```python
from build123d import *

# Parameters (mm, degrees)
SKETCH1_R           = 9
BOSS_EXTRUDE1_DEPTH = 5
CUT_EXTRUDE1_START  = -3.9
SKETCH2_R           = 9
SKETCH2_R_2         = 8
CUT_EXTRUDE1_DEPTH  = 3.9
SKETCH3_R           = 4
CUT_EXTRUDE2_DEPTH  = 5
FILLET1_R           = 0.5
FILLET2_R           = 0.1
FILLET3_R           = 0.1


with BuildPart() as part:
    # Sketch1 → Boss-Extrude1 (new body)
    with BuildSketch(Plane(origin=(0, 0, 0), x_dir=(1, 0, 0), z_dir=(0, 1, 0))):
        with Locations(Location((0, 0, 0), (0, 0, 270))):
            Circle(SKETCH1_R)
    extrude(amount=BOSS_EXTRUDE1_DEPTH)

    # Sketch2 → Cut-Extrude1 (cut)
    with BuildSketch(Plane(origin=(0, 5, 0), x_dir=(1, 0, 0), z_dir=(0, 1, 0)).offset(CUT_EXTRUDE1_START)):
        with Locations(Location((0, 0, 0), (0, 0, 270))):
            Circle(SKETCH2_R)
        with Locations(Location((0, 0, 0), (0, 0, 270))):
            Circle(SKETCH2_R_2, mode=Mode.SUBTRACT)
    extrude(amount=CUT_EXTRUDE1_DEPTH, mode=Mode.SUBTRACT)

    # Sketch3 → Cut-Extrude2 (cut)
    with BuildSketch(Plane(origin=(0, 5, 0), x_dir=(1, 0, 0), z_dir=(0, 1, 0))):
        with Locations(Location((0, 0, 0), (0, 0, 270))):
            Circle(SKETCH3_R)
    extrude(amount=-CUT_EXTRUDE2_DEPTH, mode=Mode.SUBTRACT)

    # Fillet1
    fillet1_edges = [part.edges().sort_by_distance(p)[0] for p in [
        (0, 0, -4),
        (0, 5, -4),
        (0, 5, -8),
    ]]
    fillet(fillet1_edges, radius=FILLET1_R)

    # Fillet2
    fillet2_edges = [part.edges().sort_by_distance(p)[0] for p in [
        (0, 1.1, -9),
    ]]
    fillet(fillet2_edges, radius=FILLET2_R)

    # Fillet3
    fillet3_edges = [part.edges().sort_by_distance(p)[0] for p in [
        (0, 0, -9),
    ]]
    fillet(fillet3_edges, radius=FILLET3_R)


solid = part.part
```
Design review of the part built by this model. Coordinates are the model's own, in mm. A direction names the side the tool comes from. Coordinates: 2 decimals unless noted, no trailing zeros. Order: outer loops, then holes, each group sorted by start corner. A loop starts at its lowest first (then second) coordinate and runs counter-clockwise, first axis right, second up. Notation, with made-up numbers: M -14.75,20 L 11.25,20 A23 cw 11.25,57 Z; hole C 50.25,-1.75 d3. An arc over 180 degrees is marked long. Answer as a JSON object with one key per item and string values. Group by question number.
1) Tool access review of faces 1 (the cylindrical face through (2.703, 0.544, 8.584)), 2 (the flat face through (5, 1.1, -7)): name each direction out of +Z, -Z, +X, -X, +Y, -Y from which nothing blocks a thin tool from reaching the whole face with its end or side.
2) Add section C-C, the plane y = 1.75. Write out the cut boundary in (x, z), then the cut area to 3 significant figures.
3) Wall thickness on L1, parallel to X at y = 1.7, z = 0; L2, parallel to Z at x = 1, y = 1.55; L3, parallel to X at y = 0.7, z = -2.5: over which ranges is each line inside the solid? List them lowest first.
4) Mouldability with a two-part tool opening along X and no side actions: class faces 3 (the cylindrical face through (-7.81, 2.78, -1.73)), 4 (the flat face through (-4, 0, 4)), 5 (the cylindrical face through (-3.905, 2.528, -0.867)) as pulls with the +X half, pulls with the -X half, needs draft (parallel to the pull), parting line crosses it, or undercut.
5) For pin 1 (5 mm diameter, centred on x = 0, z = 0, fed in from -Y); pin 2 (3 mm diameter, centred on y = 3.5, z = 0.5, fed in from +X); pin 3 (3 mm diameter, centred on x = 1.5, y = 3, fed in from -Z), all flat-tipped, find the tip position at first contact; note any pin that passes through.
6) Add section B-B, the plane z = 0. Write out the cut boundary in (x, y), then the cut area to 3 significant figures.
7) Add section A-A, the plane x = 0. Write out the cut boundary in (y, z).
Computed values:
{
 "1": {"face 1": "+Y, -Y", "face 2": "+Y"},
 "2": {"outline": "C 0,0 d16; hole C 0,0 d8", "area": "151 mm^2"},
 "3": {"L1": "x = -8 to -4, 4 to 8", "L2": "z = -7.94 to -3.87, 3.87 to 7.94", "L3": "x = -8.65 to -3.12, 3.12 to 8.65"},
 "4": {"face 3": "parting line crosses it", "face 4": "needs draft", "face 5": "undercut"},
 "5": {"pin 1": "passes through", "pin 2": "stops at x = 8", "pin 3": "stops at z = -8"},
 "6": {"outline": "M -9,0.1 A0.1 ccw -8.9,0 L -4.5,0 A0.5 ccw -4,0.5 L -4,4.5 A0.5 ccw -4.5,5 L -7.5,5 A0.5 ccw -8,4.5 L -8,1.1 L -8.9,1.1 A0.1 ccw -9,1 Z; M 4,0.5 A0.5 ccw 4.5,0 L 8.9,0 A0.1 ccw 9,0.1 L 9,1 A0.1 ccw 8.9,1.1 L 8,1.1 L 8,4.5 A0.5 ccw 7.5,5 L 4.5,5 A0.5 ccw 4,4.5 Z", "area": "41.9 mm^2"},
 "7": {"outline": "M 0,-8.9 A0.1 ccw 0.1,-9 L 1,-9 A0.1 ccw 1.1,-8.9 L 1.1,-8 L 4.5,-8 A0.5 ccw 5,-7.5 L 5,-4.5 A0.5 ccw 4.5,-4 L 0.5,-4 A0.5 ccw 0,-4.5 Z; M 0,4.5 A0.5 ccw 0.5,4 L 4.5,4 A0.5 ccw 5,4.5 L 5,7.5 A0.5 ccw 4.5,8 L 1.1,8 L 1.1,8.9 A0.1 ccw 1,9 L 0.1,9 A0.1 ccw 0,8.9 Z"}
}
